Design review of the part built by this model. Coordinates are the model's own, in mm. A direction names the side the tool comes from. Coordinates: 2 decimals unless noted, no trailing zeros. Loops run counter-clockwise (first coordinate to the right, second up) from the corner with the lowest first, then second, coordinate; pieces in that order, holes last. Notation, with made-up numbers: (-28.5, 45) - (8.5, 45) arc R21 cw to (8.5, 62) - close; hole circle Ø11 at (55, -5). An arc over 180 degrees is marked (long way). One line per question, with ' | ' between items.
from build123d import *

# Parameters (mm, degrees)
SKETCH_1_W                 = 23
SKETCH_1_H                 = 23
EXTRUDE_1_DEPTH            = 2
SKETCH_2_W                 = 7
SKETCH_2_H                 = 7
EXTRUDE_2_DEPTH            = 1.5
FILLET_1_R                 = 3
HOLE_WIZARD_M4_1_OUTLINE_R = 2.25
HOLE_WIZARD_M4_1_DEPTH     = 2


# Read off the part's stored shape, not the designer's step: M4 间隙孔1
with BuildPart() as part:
    # 草图1 → 凸台-拉伸1 (new body)
    with BuildSketch(Plane.XY):
        with Locations((11.5, 11.5)):
            Rectangle(SKETCH_1_W, SKETCH_1_H)
    extrude(amount=EXTRUDE_1_DEPTH)

    # 草图2 → 凸台-拉伸2 (add)
    with BuildSketch(Plane(origin=(0, 0, 0), x_dir=(-1, 0, 0), z_dir=(0, 0, -1))):
        with Locations((-11.5, 11.5)):
            Rectangle(SKETCH_2_W, SKETCH_2_H)
    extrude(amount=EXTRUDE_2_DEPTH)

    # 圆角1
    fillet_1_edges = [part.edges().sort_by_distance(p)[0] for p in [
        (0, 23, 1),
        (23, 23, 1),
        (23, 0, 1),
        (0, 0, 1),
    ]]
    fillet(fillet_1_edges, radius=FILLET_1_R)

    # M4 间隙孔1 outline → M4 间隙孔1 (cut)
    with BuildSketch(Plane.XY):
        with Locations((3.5, 3.5)):
            Circle(HOLE_WIZARD_M4_1_OUTLINE_R)
        with Locations((19.5, 19.5)):
            Circle(HOLE_WIZARD_M4_1_OUTLINE_R)
        with Locations((19.5, 3.5)):
            Circle(HOLE_WIZARD_M4_1_OUTLINE_R)
        with Locations((3.5, 19.5)):
            Circle(HOLE_WIZARD_M4_1_OUTLINE_R)
        with Locations((11.5, 11.5)):
            Circle(HOLE_WIZARD_M4_1_OUTLINE_R)
    extrude(amount=HOLE_WIZARD_M4_1_DEPTH, mode=Mode.SUBTRACT)


solid = part.part
Q1. Take a section at A-A (x = 3.5). Give the boundary of the cut face in (y, z).
Returned:
outline: (0, 0) - (1.25, 0) - (1.25, 2) - (0, 2) - close; (5.75, 0) - (17.25, 0) - (17.25, 2) - (5.75, 2) - close; (21.75, 0) - (23, 0) - (23, 2) - (21.75, 2) - close
Q2. Draft analysis for pull direction Y (two halves, no side actions). For faces 1 (the flat face through (23, 11, 1)), 2 (the cylindrical face through (3.012, 1.304, 0.986)), 3 (the cylindrical face through (22.1, 22.14, 1.01)), state which applies: +Y half, -Y half, draft (parallel to the pull), parting line (faces both ways), or undercut.
Returned:
face 1: draft | face 2: undercut | face 3: +Y half
Q3. Tool access review of faces 4 (the flat face through (12, 15, -1)), 5 (the flat face through (8, 11, -1)), 6 (the flat face through (11, 0, 1)), 7 (the cylindrical face through (9.84, 13.02, 0.99)), 8 (the flat face through (12, 8, -1)): name each direction out of +Z, -Z, +X, -X, +Y, -Y from which nothing blocks a thin tool from reaching the whole face with its end or side.
Returned:
face 4: -Z, +X, -X, +Y | face 5: -Z, -X, +Y, -Y | face 6: +Z, -Z, +X, -X, -Y | face 7: +Z | face 8: -Z, +X, -X, -Y
Q4. Take a section at C-C (z = 1). Give the boundary of the cut face in (x, y).
Returned:
outline: (0, 3) arc R3 ccw to (3, 0) - (20, 0) arc R3 ccw to (23, 3) - (23, 20) arc R3 ccw to (20, 23) - (3, 23) arc R3 ccw to (0, 20) - close; hole circle Ø4.5 at (3.5, 3.5); hole circle Ø4.5 at (3.5, 19.5); hole circle Ø4.5 at (11.5, 11.5); hole circle Ø4.5 at (19.5, 3.5); hole circle Ø4.5 at (19.5, 19.5)
Q5. To check wall thickness, follow line 1 along Y through (x, z) = (19.5, 0.55); line 2 along Y through (x, z) = (5, 1.2); line 3 along Z through (x, y) = (20.75, 12.25). State the ranges of each line that lie inside material, in increasing order.
Returned:
line 1: y = 0 to 1.25, 5.75 to 17.25, 21.75 to 23 | line 2: y = 0 to 1.82, 5.18 to 17.82, 21.18 to 23 | line 3: z = 0 to 2
Q6. Take a section at D-D (x = 11.5). Give the boundary of the cut face in (y, z), plus the area to 3 significant figures.
Returned:
outline: (0, 0) - (8, 0) - (8, -1.5) - (15, -1.5) - (15, 0) - (23, 0) - (23, 2) - (13.75, 2) - (13.75, 0) - (9.25, 0) - (9.25, 2) - (0, 2) - close | area: 47.5 mm²
Q7. For pin 1 (2.5 mm diameter, centred on x = 11.5, y = 11.5, fed in from +Z); pin 2 (4 mm diameter, centred on x = 3.5, y = 19.5, fed in from +Z) (3 decimals); pin 3 (6 mm diameter, centred on x = 19.5, y = 3.5, fed in from -Z), all flat-tipped, find the tip position at first contact; note any pin that passes through.
Returned:
pin 1: stops at z = 0 | pin 2: passes through | pin 3: stops at z = 0
